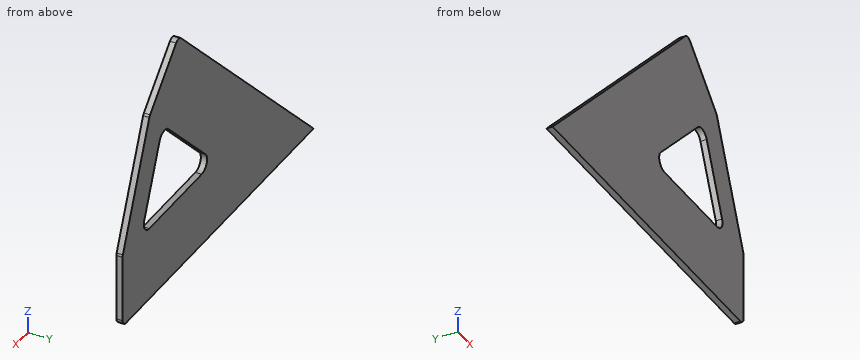
```python
from build123d import *

# Parameters (mm, degrees)
F1_DEPTH = 3.175
F2_R     = 5.08
F3_R     = 3.175


with BuildPart() as f1:
    # F0 (on Front) → F1 (new body)
    with BuildSketch(Plane.XZ):
        Polygon((41.632985, 114.545227), (-84.090601, -11.178358), (93.709399, -11.178358), (93.709399, 26.921642), (68.573753, 87.604459), align=None)
        Polygon((7.890936, 26.921642), (56.423554, 75.45426), (76.526423, 26.921642), align=None, mode=Mode.SUBTRACT)
    extrude(amount=F1_DEPTH)

    # F2
    f2_edges = [f1.edges().sort_by_distance(p)[0] for p in [
        (7.890936, -1.5875, 26.921642),
        (76.526423, -1.5875, 26.921642),
        (56.423554, -1.5875, 75.45426),
    ]]
    fillet(f2_edges, radius=F2_R)

    # F3
    f3_edges = [f1.edges().sort_by_distance(p)[0] for p in [
        (41.632985, -1.5875, 114.545227),
        (68.573753, -1.5875, 87.604459),
        (93.709399, -1.5875, 26.921642),
        (93.709399, -1.5875, -11.178358),
    ]]
    fillet(f3_edges, radius=F3_R)


solid = f1.part
```
Can you work these out from the model? Positions are in its coordinate system, mm. Give positions to 0.01 mm unless a question says otherwise; leave off trailing zeros. Loops run counter-clockwise (first coordinate to the right, second up) from the corner with the lowest first, then second, coordinate; pieces in that order, holes last. Notation, with made-up numbers: M 48.25,39.5 L 54.25,39.5 A12 ccw 54.25,45.5 Z; hole C 85,82.25 d6. An arc over 180 degrees is marked long. One line per item, written item: value.
(1) Suppose I cut it at B-B on z = 56. List the corners of the cut face in (x, y) for me (3 decimals), plus the area to 3 significant figures.
Returned:
outline: M -16.912,-3.175 L 36.969,-3.175 L 36.969,0 L -16.912,0 Z; M 64.482,-3.175 L 81.665,-3.175 L 81.665,0 L 64.482,0 Z
area: 226 mm^2
(2) Suppose I cut it at D-D on x = -36.5. List the corners of the cut face in (y, z) for me (3 decimals), plus the area to 3 significant figures.
Returned:
outline: M -3.175,-11.178 L 0,-11.178 L 0,36.412 L -3.175,36.412 Z
area: 151 mm^2
(3) Suppose I cut it at A-A on y = -1.85. List the corners of the cut face in (x, z) for me (3 decimals), plus the area to 3 significant figures.
Returned:
outline: M -84.091,-11.178 L 90.534,-11.178 A3.175 ccw 93.709,-8.003 L 93.709,26.29 A3.175 ccw 93.468,27.505 L 68.815,87.021 A3.175 ccw 68.127,88.051 L 43.878,112.3 A3.175 ccw 39.388,112.3 Z; hole M 16.563,35.594 A5.08 ccw 20.155,26.922 L 68.924,26.922 A5.08 ccw 73.617,33.946 L 59.333,68.43 A5.08 ccw 51.048,70.078 Z
area: 11,000 mm^2
(4) I need wall thicknesses on line 1 (X direction, y = -2.75, z = 61.5); line 2 (Z direction, x = 30.5, y = -0.85); line 3 (Z direction, x = 65, y = -2.25). Which ranges of each line are inside material? Lowest first, please.
Returned:
line 1: -11.41 to 42.47, 62.2 to 79.39
line 2: -11.18 to 26.92, 49.53 to 103.41
line 3: -11.18 to 26.92, 54.75 to 91.18
(5) Suppose I cut it at C-C on x = 62. List the corners of the cut face in (y, z) for me (3 decimals), plus the area to 3 significant figures.
Returned:
outline: M -3.175,-11.178 L 0,-11.178 L 0,26.922 L -3.175,26.922 Z; M -3.175,61.992 L 0,61.992 L 0,94.178 L -3.175,94.178 Z
area: 223 mm^2
(6) Will this pin go through, and if not, where does the flat tip stop? pin 1 (1.5 mm diameter, centred on y = -3, z = 52.5, fed in from -X).
Returned:
pin 1: x = -21.16
